Model file for the job. Use its own axes, mm. Face numbers are marked on the shaded views. A direction names the side the tool comes from. Round coordinates to 2 decimals unless told otherwise and drop trailing zeros. Loops run counter-clockwise (first coordinate to the right, second up) from the corner with the lowest first, then second, coordinate; pieces in that order, holes last. Notation, with made-up numbers: (79.25, -33.75) -> (94.25, -33.75) arc R23 ccw to (94.25, 2.25) -> close; hole circle Ø8 at (-40, -16). An arc over 180 degrees is marked (long way). Use a Markdown table: item, result.
Autodesk Inventor part; units mm, degrees
ref_plane "YZ Plane" through (0, 0, 0) normal (1, 0, 0) x (0, 1, 0)
ref_plane "XZ Plane" through (0, 0, 0) normal (0, 1, 0) x (-1, 0, 0)
ref_plane "XY Plane" through (0, 0, 0) normal (0, 0, 1) x (1, 0, 0)
sketch "Sketch1" plane through (0, 0, 0) normal (0, 1, 0) x (-1, 0, 0)
  circle A0 centre (0, 0) radius 1.4
  dimension "d0" = 2.8
sketch "Sketch2" plane through (0, 0, 0) normal (0, 1, 0) x (-1, 0, 0)
  point P0 (0, 0)
extrude "Extrusion1" add sketch "Sketch1" along normal blind 7
sketch "Sketch3" plane through (0, 7, 0) normal (0, 1, 0) x (1, 0, 0)
  line L0 (1.8253, 0.7457) -> (1.818, -0.7634)
  line L1 (1.818, -0.7634) -> (0.7457, -1.8253)
  line L2 (0.7457, -1.8253) -> (-0.7634, -1.818)
  line L3 (-0.7634, -1.818) -> (-1.8253, -0.7457)
  line L4 (-1.8253, -0.7457) -> (-1.818, 0.7634)
  line L5 (-1.818, 0.7634) -> (-0.7457, 1.8253)
  line L6 (-0.7457, 1.8253) -> (0.7634, 1.818)
  line L7 (0.7634, 1.818) -> (1.8253, 0.7457)
  line L8 (-1.8216, 0.0088) -> (1.8216, -0.0088) construction
  line L9 (-0.0088, -1.8216) -> (0.0088, 1.8216) construction
  point P0 (0, 0)
  point P1 (0, 0)
  point P2 (0, 0)
  point P3 (0, 0)
extrude "Extrusion2" add sketch "Sketch3" along normal blind 2
sketch "Sketch4" plane through (-0.7457, 7, -1.8253) normal (0.0049, 0, -1) x (-1, 0, -0.0049)
  line L0 (-1.5091, 2) -> (0, 2)
  line L1 (0, 2) -> (0, 0)
  line L2 (0, 0) -> (-1.5091, 0)
  line L3 (-1.5091, 0) -> (-1.5091, 2)
  point P0 (-0.7546, -7)
extrude "Extrusion3" add sketch "Sketch4" along normal blind 10
sketch "Sketch5" plane through (0, 9, 0) normal (0, 1, 0) x (1, 0, 0)
  point P0 (0, 0)
sketch "Sketch6" plane through (0, 9, 0) normal (0, 1, 0) x (1, 0, 0)
  point P0 (0, 0)
thread "Thread1"
sketch "Sketch7" plane through (0, 9, 0) normal (0, 1, 0) x (1, 0, 0)
  circle A0 centre (0.062, 12.7642) radius 1.2414
  point P0 (0, 0)
extrude "Extrusion4" add sketch "Sketch7" against normal blind 2
sketch "Sketch8" plane through (0, 9, 0) normal (0, 1, 0) x (1, 0, 0)
  point P0 (0, 0)
sketch "Sketch9" plane through (0, 9, 0) normal (0, 1, 0) x (1, 0, 0)
  point P0 (0, 0)
sketch "Sketch10" plane through (0, 9, 0) normal (0, 1, 0) x (1, 0, 0)
  line L0 (0.8117, 11.7749) -> (0.8213, 13.7463)
  arc A0 (0.8117, 11.7749) -> (-0.6974, 11.7822) centre (0.062, 12.7642) ccw
  line L1 (0.7634, 1.818) -> (0.8117, 11.7749)
  line L2 (0.8213, 13.7463) -> (10.3239, 13.7463)
  line L3 (10.3239, 13.7463) -> (10.3239, 11.7749)
  line L4 (10.3239, 11.7749) -> (0.8117, 11.7749)
  line L5 (5.5726, 13.7463) -> (5.5678, 11.7749) construction
  arc A1 (11.8329, 11.7518) -> (10.3238, 11.7518) centre (11.0784, 12.7375) ccw
  arc A2 (10.3238, 11.7518) -> (11.8329, 11.7518) centre (11.0784, 12.7375) ccw
  point P0 (0, 0)
extrude "Extrusion5" add sketch "Sketch10" against normal blind 4 contours A0 L2 L3 A1 L4 | A1 L3 L4
sketch "Sketch11" plane through (0, 9, 0) normal (0, 1, 0) x (1, 0, 0)
  point P0 (0, 0)
properties part number "Servo_Arm_Hook"
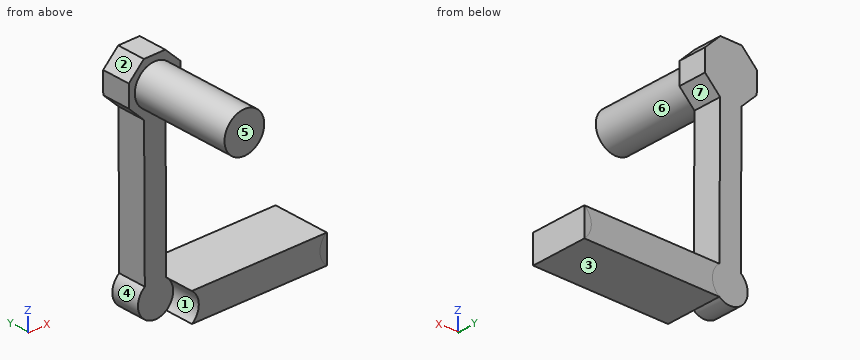
Q1. Tool access for the marked faces 5, 6 and 7: list every direction of +Z, -Z, +X, -X, +Y, -Y with a clear straight run to the whole face (end or side of a thin tool).
Results list:
| item | result |
|---|---|
| face 5 | +Z, -Z, +X, -X, -Y |
| face 6 | -Y |
| face 7 | +X, +Y, -Y |
Q2. Band-saw the part on C-C, the plane z = 0. Give the cut face in (x, y).
Results list:
| item | result |
|---|---|
| outline | (-1.82, 7) -> (-1.4, 7) -> (-1.4, 0) -> (1.4, 0) -> (1.4, 7) -> (1.82, 7) -> (1.82, 9) -> (-1.82, 9) -> close |
Q3. Drill centre lines: L1, parallel to Z at x = 4.75, y = 6.5; L2, parallel to Y at x = -0.25, z = -12.5; L3, parallel to Z at x = 0, y = 2.5. Where is each one in solid material? Low to high. Write a range as from..to.
Results list:
| item | result |
|---|---|
| L1 | z = -13.75..-11.77 |
| L2 | y = 7..9 |
| L3 | z = -1.4..1.4 |
Q4. Band-saw the part on D-D, the plane x = 8.5. Give the cut face in (y, z), plus the area to 3 significant figures.
Results list:
| item | result |
|---|---|
| outline | (5, -13.75) -> (9, -13.75) -> (9, -11.77) -> (5, -11.77) -> close |
| area | 7.89 mm² |
Q5. Pull direction Z, two halves, no side cores. Call the marked faces 1, 2, 3 and 4: released by +Z, released by -Z, zero draft, split by the parting line, or undercut.
Results list:
| item | result |
|---|---|
| face 1 | undercut |
| face 2 | released by +Z |
| face 3 | released by -Z |
| face 4 | undercut |
Q6. Flat gauge pins, fed straight in: pin 1 (1.2 mm diameter, centred on x = 5.5, y = 7, fed in from +Z); pin 2 (0.5 mm diameter, centred on x = 10, z = -12.5, fed in from -Y); pin 3 (4.5 mm diameter, centred on x = 5, y = 7.5, fed in from -Z); pin 4 (4 mm diameter, centred on x = 0, y = 7.5, fed in from +Z). Where does each tip first touch, or does it go through?
Results list:
| item | result |
|---|---|
| pin 1 | stops at z = -11.77 |
| pin 2 | stops at y = 5 |
| pin 3 | stops at z = -13.75 |
| pin 4 | stops at z = 1.83 |
Q7. Band-saw the part on A-A, the plane x = -1. Give the cut face in (y, z), plus the area to 3 significant figures.
Results list:
| item | result |
|---|---|
| outline | (0, -0.98) -> (7, -0.98) -> (7, -1.57) -> (9, -1.57) -> (9, 1.58) -> (7, 1.58) -> (7, 0.98) -> (0, 0.98) -> close; (7, -13.41) -> (9, -13.41) -> (9, -12.12) -> (7, -12.12) -> close |
| area | 22.6 mm² |
